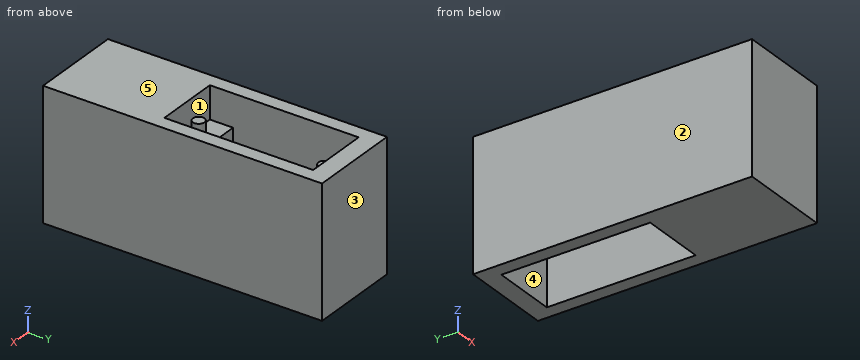
Autodesk Fusion 360 part; units mm, degrees
sketch "Sketch1" plane through (0, 0, 0) normal (0, 0, 1) x (1, 0, 0) in component "Elbow"
  line L0 (10, 30) -> (-10, 30)
  line L1 (-10, 30) -> (-10, -30)
  line L2 (-10, -30) -> (10, -30)
  line L3 (10, -30) -> (10, 30)
  line L4 (10, 30) -> (-10, -30) construction
  line L5 (-10, 30) -> (10, -30) construction
  line L6 (7, 26) -> (-7, 26)
  line L7 (-7, 26) -> (-7, -6)
  line L8 (-7, -6) -> (7, -6)
  line L9 (7, -6) -> (7, 26)
  line L10 (7, 26) -> (-7, -6) construction
  line L11 (-7, 26) -> (7, -6) construction
  point P0 (0, 10)
extrude "Extrude1" add sketch "Sketch1" along normal blind 28 in component "Elbow"
sketch "Sketch2" plane through (0, 0, 0) normal (0, 0, 1) x (1, 0, 0) in component "Elbow"
  line L0 (-7, -6) -> (7, -6)
  line L1 (7, -6) -> (7, -1)
  line L2 (7, -1) -> (-7, -1)
  line L3 (-7, -1) -> (-7, -6)
  line L4 (-7, 26) -> (7, 26)
  line L5 (7, 26) -> (7, 21)
  line L6 (7, 21) -> (-7, 21)
  line L7 (-7, 21) -> (-7, 26)
extrude "Extrude2" add sketch "Sketch2" along normal blind 21 in component "Elbow"
sketch "Sketch3" plane through (0, 0, 0) normal (0, 0, 1) x (1, 0, 0) in component "Elbow"
  line L0 (-7, -1) -> (7, -1)
  line L1 (7, -1) -> (7, -6)
  line L2 (7, -6) -> (-7, -6)
  line L3 (-7, -6) -> (-7, -1)
  line L4 (-7, 26) -> (7, 26)
  line L5 (7, 26) -> (7, 21)
  line L6 (7, 21) -> (-7, 21)
  line L7 (-7, 21) -> (-7, 26)
extrude "Extrude3" cut sketch "Sketch3" along normal blind 16 in component "Elbow"
sketch "Sketch4" plane through (0, 0, 21) normal (0, 0, 1) x (-1, 0, 0) in component "Elbow"
  line L0 (7, 1) -> (7, 6)
  line L1 (7, 6) -> (-7, 6)
  line L2 (-7, 6) -> (-7, 1)
  line L3 (-7, 1) -> (7, 1)
  circle A0 centre (0, 3.5) radius 1.25
  dimension "d7" = 2.5
extrude "Extrude4" add sketch "Sketch4" along normal blind 4 contours A0 in component "Elbow"
sketch "Sketch5" plane through (0, 0, 21) normal (0, 0, 1) x (-1, 0, 0) in component "Elbow"
  line L0 (7, -21) -> (-7, -21)
  line L1 (-7, -21) -> (-7, -26)
  line L2 (-7, -26) -> (7, -26)
  line L3 (7, -26) -> (7, -21)
  circle A0 centre (0, -23.5) radius 1.25
  dimension "d10" = 2.5
extrude "Extrude5" add sketch "Sketch5" along normal blind 4 contours A0 in component "Elbow"
component "Elbow" placed x (1, 0, 0) y (0, 1, 0) z (0, 0, 1) at (0, 0, 0)
Source: CAD feature listing. Evaluate the final solid. Frame: model axes, mm. Face numbers are marked on the shaded views. A direction names the side the tool comes from. Give positions to 0.01 mm unless a question says otherwise; leave off trailing zeros. Write each loop counter-clockwise with the first axis right and the second up, starting at its lowest first coordinate (ties: lowest second). Pieces come first, ordered by that corner, then holes. Notation, with made-up numbers: (23.25, -31) -> (56.25, -31) arc R29 ccw to (56.25, 4) -> close; hole circle Ø5 at (-30, 10.25). An arc over 180 degrees is marked (long way). Write item = value, one per line.
Q1. Mould query, pull axis X, two halves, no side actions, for the marked faces 1, 2 and 3. Classes: +X half, -X half, draft (parallel to the pull), parting line (faces both ways), or undercut.
Here are the results:
face_1 = undercut
face_2 = -X half
face_3 = draft
Q2. Cut plane D-D on z = 9.25. Return loops of the section in (x, y).
Here are the results:
outline = (-10, -30) -> (10, -30) -> (10, 30) -> (-10, 30) -> close; hole (-7, -6) -> (7, -6) -> (7, 26) -> (-7, 26) -> close
Q3. First-contact query: pin 1 (2.5 mm diameter, centred on x = 0, y = 24.5, fed in from -Z); pin 2 (1.2 mm diameter, centred on x = 0.5, y = -3.5, fed in from +Z). Flat tips, straight axial feed; report the tip coordinate or a pass-through.
Here are the results:
pin_1 = 16
pin_2 = 25
Q4. Cut plane C-C on y = 8. Return loops of the section in (x, z).
Here are the results:
outline = (-10, 0) -> (-7, 0) -> (-7, 28) -> (-10, 28) -> close; (7, 0) -> (10, 0) -> (10, 28) -> (7, 28) -> close
Q5. Cut plane B-B on x = 0. Return loops of the section in (y, z), then the cut area to 3 significant figures.
Here are the results:
outline = (-30, 0) -> (-6, 0) -> (-6, 16) -> (-1, 16) -> (-1, 21) -> (-2.25, 21) -> (-2.25, 25) -> (-4.75, 25) -> (-4.75, 21) -> (-6, 21) -> (-6, 28) -> (-30, 28) -> close; (21, 16) -> (26, 16) -> (26, 0) -> (30, 0) -> (30, 28) -> (26, 28) -> (26, 21) -> (24.75, 21) -> (24.75, 25) -> (22.25, 25) -> (22.25, 21) -> (21, 21) -> close
area = 854 mm²
Q6. Cut plane A-A on z = 23. Return loops of the section in (x, y), then the cut area to 3 significant figures.
Here are the results:
outline = (-10, -30) -> (10, -30) -> (10, 30) -> (-10, 30) -> close; circle Ø2.5 at (0, -3.5); circle Ø2.5 at (0, 23.5); hole (-7, -6) -> (7, -6) -> (7, 26) -> (-7, 26) -> close
area = 762 mm²
Q7. Reachability of the marked faces 4 and 5 from +Z, -Z, +X, -X, +Y, -Y: full face, straight path, thin tool, end or side. Return the list, or none.
Here are the results:
face_4 = -Z
face_5 = +Z, +X, -X, +Y, -Y
Q8. Line query: line 1 (X direction, y = 0, z = 17.75); line 2 (Y direction, x = -0.5, z = 11.75); line 3 (Y direction, x = 5.25, z = 18.5). Output: solid intervals per line, ascending. Write a range as from..to.
Here are the results:
line_1 = -10..-7, 7..10
line_2 = -30..-6, 26..30
line_3 = -30..-1, 21..30
